Could you check a few things on this model? Use its own coordinates, in mm. Face numbers are marked on the shaded views. A direction names the side the tool comes from. Coordinates: 2 decimals unless noted, no trailing zeros. Write each loop counter-clockwise with the first axis right and the second up, starting at its lowest first coordinate (ties: lowest second). Pieces come first, ordered by that corner, then holes. Notation, with made-up numbers: M -16.5,74.25 L 22.5,74.25 A29 ccw 22.5,111.25 Z; hole C 6,44.5 d4. An arc over 180 degrees is marked long. Answer as CSV lines item,"result". Start each with the question number.
Item 1: I'm going to push flat-ended pins straight in: P1, Ø2, axis at x = 81.5, z = 33.5, coming from the +Y side; P2, Ø3, axis at y = 4, z = 54, coming from the +X side; P3, Ø6, axis at x = 53, z = 48, coming from the +Y side; P4, Ø2.5, axis at y = 24, z = 21, coming from the -X side. Where does each tip first touch, or does it pass through?
Item 2: On a 3-axis mill with a long thin cutter (end or side, diameter ignored), from which of +Z, -Z, +X, -X, +Y, -Y can I reach the whole of each face in a straight line? I mean the marked faces 4, 5 and 6. Say none if no direction works.
Item 3: Suppose I cut it at C-C, the plane x = 43. Write out the boundary of the cut face in (y, z).
Item 4: Suppose I cut it at D-D, the plane z = 46. Write out the boundary of the cut face in (x, y), and give its area (3 significant figures).
Item 5: If I drill on line 1 along Z through (x, y) = (85, 7.1); line 2 along Z through (x, y) = (85, 1.2); line 3 along Z through (x, y) = (58.5, 20.5), over which ranges is the centre line in solid material (lowest first)? Write a range as [from, to].
Item 6: Suppose I cut it at A-A, the plane x = 31.5. Write out the boundary of the cut face in (y, z).
Item 7: We'd pull the mould along Y, two halves only. Please class the marked faces 1, 2 and 3: +Y half, -Y half, draft (parallel to the pull), parting line (faces both ways), or undercut.
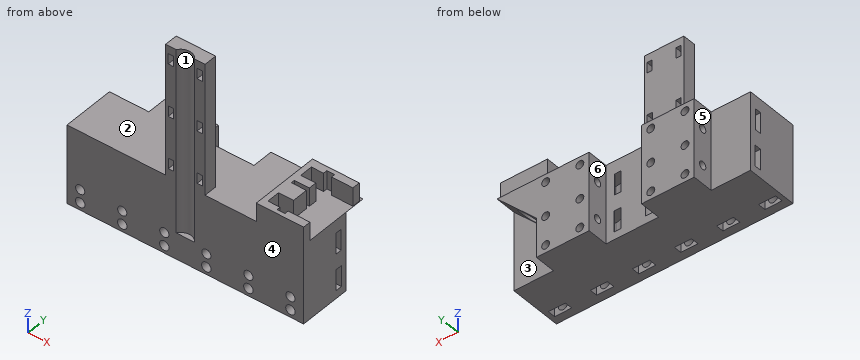
```python
from build123d import *

# Parameters (mm, degrees)
F1_DEPTH  = 30
F3_W      = 2.5
F3_H      = 8
F5_W      = 2.5
F5_H      = 8
F8_R      = 1.811637
F8_R_2    = 1.75
F10_DEPTH = 10
F9_W      = 6.5
F9_H      = 3
F11_DEPTH = 12
F12_R     = 1.5
F13_DEPTH = 20
F14_W     = 15
F14_H     = 5
F15_DEPTH = 50
F17_DEPTH = 70
F18_W     = 2
F18_H     = 4
F19_DEPTH = 28.001
F22_DEPTH = 8
F7_R      = 1.5
F23_DEPTH = 75.001
F24_R     = 3.5
F25_DEPTH = 15
F26_DEPTH = 7


with BuildPart() as f1:
    # F0 (on Top) → F1 (new body)
    with BuildSketch(Plane.XY):
        Polygon((0, 20), (0, 0), (90, 0), (90, 20), (75, 20), (75, 28), (55, 28), (55, 20), (35, 20), (35, 28), (15, 28), (15, 20), align=None)
    extrude(amount=F1_DEPTH)

    # F4: sweep along a path in F2
    with BuildLine(Plane.XY.offset(30)) as f4_path:
        Line((0, 16.5), (35, 16.5))
        ThreePointArc((35, 16.5), (37.780873, 17.683526), (38.855914, 20.508111))
    # F3 (on face) → F4 (sweep, cut)
    with BuildSketch(Plane(origin=(0, 0, 0), x_dir=(0, -1, 0), z_dir=(-1, 0, 0))):
        with Locations((-16.5, 21)):
            Rectangle(F3_W, F3_H)
        with Locations((-16.550689, 7)):
            Rectangle(F3_W, F3_H)
    sweep(path=f4_path.line, mode=Mode.SUBTRACT)

    # F6: sweep along a path in F2
    with BuildLine(Plane.XY.offset(30)) as f6_path:
        Line((90, 16.5), (55, 16.5))
        ThreePointArc((55, 16.5), (51.896558, 17.690089), (50.384562, 20.650078))
    # F5 (on face) → F6 (sweep, cut)
    with BuildSketch(Plane.YZ.offset(90)):
        with Locations((16.5, 21)):
            Rectangle(F5_W, F5_H)
        with Locations((16.589286, 7)):
            Rectangle(F5_W, F5_H)
    sweep(path=f6_path.line, mode=Mode.SUBTRACT)

    # F8 (on face) → F10 (cut)
    with BuildSketch(Plane.XZ):
        with Locations((5, 2.839677)):
            Circle(F8_R)
        with Locations((5, 7.839677)):
            Circle(F8_R_2)
        with Locations((21, 7.839677)):
            Circle(F8_R_2)
        with Locations((21, 2.839677)):
            Circle(F8_R)
        with Locations((37, 7.839677)):
            Circle(F8_R_2)
        with Locations((37, 2.839677)):
            Circle(F8_R)
        with Locations((53, 7.839677)):
            Circle(F8_R_2)
        with Locations((53, 2.839677)):
            Circle(F8_R)
        with Locations((69, 7.839677)):
            Circle(F8_R_2)
        with Locations((69, 2.839677)):
            Circle(F8_R)
        with Locations((85, 7.839677)):
            Circle(F8_R_2)
        with Locations((85, 2.839677)):
            Circle(F8_R)
    extrude(amount=-F10_DEPTH, mode=Mode.SUBTRACT)

    # F9 (on face) → F11 (cut)
    with BuildSketch(Plane(origin=(0, 0, 0), x_dir=(1, 0, 0), z_dir=(0, 0, -1))):
        with Locations((5, -4.5)):
            Rectangle(F9_W, F9_H)
        with Locations((21, -4.5)):
            Rectangle(F9_W, F9_H)
        with Locations((37, -4.5)):
            Rectangle(F9_W, F9_H)
        with Locations((53, -4.5)):
            Rectangle(F9_W, F9_H)
        with Locations((69, -4.5)):
            Rectangle(F9_W, F9_H)
        with Locations((85, -4.5)):
            Rectangle(F9_W, F9_H)
    extrude(amount=-F11_DEPTH, mode=Mode.SUBTRACT)

    # F12 (on face) → F13 (cut)
    with BuildSketch(Plane(origin=(0, 28, 0), x_dir=(-1, 0, 0), z_dir=(0, 1, 0))):
        with Locations((-71.5, 27)):
            Circle(F12_R)
        with Locations((-58.5, 27)):
            Circle(F12_R)
        with Locations((-71.5, 14)):
            Circle(F12_R)
        with Locations((-58.5, 14)):
            Circle(F12_R)
        with Locations((-71.5, 3)):
            Circle(F12_R)
        with Locations((-58.5, 3)):
            Circle(F12_R)
        with Locations((-31.5, 3)):
            Circle(F12_R)
        with Locations((-18.5, 3)):
            Circle(F12_R)
        with Locations((-18.5, 14)):
            Circle(F12_R)
        with Locations((-31.5, 14)):
            Circle(F12_R)
        with Locations((-31.5, 27)):
            Circle(F12_R)
        with Locations((-18.5, 27)):
            Circle(F12_R)
    extrude(amount=-F13_DEPTH, mode=Mode.SUBTRACT)

    # F14 (on face) → F15 (join)
    with BuildSketch(Plane.XY.offset(30)):
        with Locations((45, 2.5)):
            Rectangle(F14_W, F14_H)
    extrude(amount=F15_DEPTH)

    # F16 (on face) → F17 (cut)
    with BuildSketch(Plane.XY.offset(80)):
        with BuildLine():
            Line((41.5, 0), (48.5, 0))
            ThreePointArc((48.5, 0), (45, 1.907092), (41.5, 0))
        make_face()
    extrude(amount=-F17_DEPTH, mode=Mode.SUBTRACT)

    # F18 (on face) → F19 (cut, through all)
    with BuildSketch(Plane.XZ):
        with Locations((39.5, 75)):
            Rectangle(F18_W, F18_H)
        with Locations((39.513543, 55.000005)):
            Rectangle(F18_W, F18_H)
        with Locations((39.527086, 35.000009)):
            Rectangle(F18_W, F18_H)
        with Locations((50.5, 75)):
            Rectangle(F18_W, F18_H)
        with Locations((50.486457, 55.000005)):
            Rectangle(F18_W, F18_H)
        with Locations((50.472914, 35.000009)):
            Rectangle(F18_W, F18_H)
    extrude(amount=-F19_DEPTH, mode=Mode.SUBTRACT)

    # F21 (on face) → F22 (join)
    with BuildSketch(Plane(origin=(0, 20, 0), x_dir=(-1, 0, 0), z_dir=(0, 1, 0))):
        Polygon((-75, 30), (-90, 30), (-75, 15), align=None)
    extrude(amount=F22_DEPTH)

    # F7 (on face) → F23 (cut, through all)
    with BuildSketch(Plane(origin=(15, 0, 0), x_dir=(0, -1, 0), z_dir=(-1, 0, 0))):
        with Locations((-24, 21)):
            Circle(F7_R)
        with Locations((-24, 7)):
            Circle(F7_R)
    extrude(amount=-F23_DEPTH, mode=Mode.SUBTRACT)

    # F24 (on face) → F25 (cut)
    with BuildSketch(Plane.YZ.offset(90)):
        with Locations((24.02541, 20.994468)):
            Circle(F24_R)
    extrude(amount=-F25_DEPTH, mode=Mode.SUBTRACT)

    # F20 (on face) → F26 (join)
    with BuildSketch(Plane.XY.offset(30)):
        Polygon((81.69346, 24.958679), (81.69346, 23.5), (89.806349, 23.5), (89.806349, 26.5), (72, 26.5), (72, 0), (90, 0), (90, 3), (81.69346, 3), (81.69346, 1.496212), (78.730785, 1.496212), (78.730785, 2.889788), (74.089549, 2.889788), (74.089549, 7.889788), (79.806349, 7.889788), (79.806349, 13.933841), (74.089549, 13.933841), (74.089549, 15.378134), (79.806349, 15.378134), (79.806349, 18.389788), (74.089549, 18.389788), (74.089549, 23.389788), (78.730785, 23.389788), (78.730785, 24.958679), align=None)
    extrude(amount=F26_DEPTH)


solid = f1.part
```
Ans:
1,P1,"stops at y = 26.5"
1,P2,"stops at x = 52.5"
1,P3,"stops at y = 5"
1,P4,"passes through"
2,face 4,"+Z, -Z, +X, -X, -Y"
2,face 5,"+Z, -Z, -X, +Y"
2,face 6,"+Z, -Z, +Y"
3,outline,"M 0,0 L 20,0 L 20,30 L 5,30 L 5,80 L 1.4,80 L 1.4,10 L 0,10 Z"
4,outline,"M 37.5,0 L 41.5,0 A4.17 cw 48.5,0 L 52.5,0 L 52.5,5 L 37.5,5 Z"
4,area,"65.6 mm^2"
5,line 1,"z = [0, 1.03], [4.65, 6.09], [9.59, 30]"
5,line 2,"z = [0, 1.03], [4.65, 6.09], [9.59, 37]"
5,line 3,"z = [0, 1.5], [4.5, 12.5], [15.5, 25.5], [28.5, 30]"
6,outline,"M 0,0 L 28,0 L 28,1.5 L 8,1.5 L 8,4.5 L 15.3,4.5 L 15.3,11 L 17.8,11 L 17.8,4.5 L 28,4.5 L 28,12.5 L 8,12.5 L 8,15.5 L 28,15.5 L 28,25.5 L 8,25.5 L 8,28.5 L 28,28.5 L 28,30 L 0,30 Z; hole M 15.25,17 L 17.75,17 L 17.75,25 L 15.25,25 Z; hole C 24,7 d3; hole C 24,21 d3"
7,face 1,"-Y half"
7,face 2,"undercut"
7,face 3,"+Y half"
